Autodesk Inventor part; units mm, degrees
ref_plane "YZ Plane" through (0, 0, 0) normal (1, 0, 0) x (0, 1, 0)
ref_plane "XZ Plane" through (0, 0, 0) normal (0, 1, 0) x (-1, 0, 0)
ref_plane "XY Plane" through (0, 0, 0) normal (0, 0, 1) x (1, 0, 0)
sketch "Эскиз1" plane through (0, 0, 0) normal (0, 1, 0) x (-1, 0, 0)
  line L0 (0, 0) -> (-10, 0)
  line L1 (-10, 0) -> (-10, -11)
  line L2 (-10, -11) -> (0, -11)
  line L3 (0, -11) -> (0, 0)
  dimension "d0" = 10
  dimension "d1" = 11
extrude "Выдавливание1" add sketch "Эскиз1" along normal mid plane 10
sketch "Эскиз2" plane through (0, 0, 0) normal (0, 1, 0) x (-1, 0, 0)
  line L0 (0, -11) -> (0, 0)
  line L1 (0, -5.5) -> (-10, -5.5)
  line L2 (-10, 0) -> (-10, -11)
  line L3 (-1.5, -1.5) -> (-8.5, -1.5)
  line L4 (-8.5, -1.5) -> (-8.5, -9.5)
  line L5 (-8.5, -9.5) -> (-1.5, -9.5)
  line L6 (-1.5, -9.5) -> (-1.5, -1.5)
  line L7 (-1.5, -1.5) -> (-8.5, -9.5) construction
  line L8 (-8.5, -1.5) -> (-1.5, -9.5) construction
  point P0 (-5, -5.5)
  dimension "d4" = 7
  dimension "d5" = 8
extrude "Выдавливание2" cut sketch "Эскиз2" along normal mid plane 7
fillet "Сопряжение1" radius 1 12 edges at (10, 5, -5.5) (5, -5, 0) (5, 5, 0) (0, 5, -5.5) (0, 0, 0) (0, -5, -5.5) (0, 0, -11) (10, 0, -11) (5, 5, -11) (5, -5, -11) (10, -5, -5.5) (10, 0, 0)
sketch "Эскиз3" plane through (0, -4, -1) normal (-1, 0, 0) x (0, 0, 1)
  line L0 (0, 0) -> (0, 8)
  line L1 (0, 4) -> (-9, 4)
  line L2 (-9, 0) -> (-9, 8)
  line L3 (-1, 5) -> (-8, 5)
  line L4 (-8, 5) -> (-8, 3)
  line L5 (-8, 3) -> (-1, 3)
  line L6 (-1, 3) -> (-1, 5)
  line L7 (-1, 5) -> (-8, 3) construction
  line L8 (-8, 5) -> (-1, 3) construction
  point P0 (1, 4)
  point P1 (-4.5, 4)
sketch "Эскиз6" plane through (10, -4, -1) normal (1, 0, 0) x (0, 0, -1)
  line L0 (1, 3) -> (8, 3)
  line L1 (1, 5) -> (1, 3)
  line L2 (8, 5) -> (1, 5)
  line L3 (8, 3) -> (8, 5)
  point P0 (-1, 4)
sketch "Эскиз7" plane through (0, 5, 0) normal (0, 1, 0) x (1, 0, 0)
  line L0 (9, 1) -> (1, 1)
  line L1 (5, 1) -> (5, 10)
  line L2 (9, 10) -> (1, 10)
  line L3 (4, 2) -> (6, 2)
  line L4 (6, 2) -> (6, 9)
  line L5 (6, 9) -> (4, 9)
  line L6 (4, 9) -> (4, 2)
  line L7 (4, 2) -> (6, 9) construction
  line L8 (6, 2) -> (4, 9) construction
  point P0 (0, 0)
  point P1 (5, 5.5)
sketch "Эскиз8" plane through (0, -5, 0) normal (0, -1, 0) x (1, 0, 0)
  line L0 (4, -9) -> (4, -2)
  line L1 (6, -9) -> (4, -9)
  line L2 (6, -2) -> (6, -9)
  line L3 (4, -2) -> (6, -2)
  point P0 (0, 0)
extrude "Выдавливание5" cut sketch "Эскиз7" against normal blind 0.5
extrude "Выдавливание6" cut sketch "Эскиз3" against normal blind 0.5
extrude "Выдавливание7" cut sketch "Эскиз8" against normal blind 0.5
extrude "Выдавливание8" cut sketch "Эскиз6" against normal blind 0.5
properties part number "cube"
The listing builds one solid part. Answer for the finished solid, in the listing's coordinates (mm). A direction names the side the tool comes from. Give positions to 0.01 mm unless a question says otherwise; leave off trailing zeros. Write each loop counter-clockwise with the first axis right and the second up, starting at its lowest first coordinate (ties: lowest second). Pieces come first, ordered by that corner, then holes. Notation, with made-up numbers: (21, 43.5) - (28, 43.5) arc R29 cw to (28, 77.5) - close; hole circle Ø10 at (-20, 39). An arc over 180 degrees is marked (long way). Use one line per item in the form item = value. Start each with the question number.
1) The mould has two halves that part along Z. Classify faces 1 (the face through (0.285, -4.699, -5.437)), 2 (the face through (0.5, 0, -6)), 3 (the face through (9.699, 0.056, -0.285)), 4 (the face through (5, 0, -11)): pulls with the +Z half, pulls with the -Z half, needs draft (parallel to the pull), parting line crosses it, or undercut.
2) Consider line 1 along X through (y, z) = (1, -9.25); line 2 along Z through (x, y) = (4, -2); line 3 along Y through (x, z) = (7.25, -5.5). Determine where each line is inside the solid, lowest interval first. Write a range as from..to.
3) Flat-ended cylindrical pins translate along their axes: pin 1 Ø2 at (x, z) = (4.5, -7) entering from -Y; pin 2 Ø0.6 at (x, z) = (0.5, -4) entering from +Y. Find the tip coordinate at first contact, or state that the pin passes through.
4) Find section C-C on z = -3.5. Determine the outline of the cut face in (x, y), plus the area to 3 significant figures.
5) A tool of negligible diameter and unlimited length cuts with its end or side. For faces 5 (the face through (4.944, 4.715, -10.699)), 6 (the face through (5, 4.5, -6)), 7 (the face through (5, -3.5, -5)), 8 (the face through (9.715, -4.699, -5.563)), 9 (the face through (5, -4.5, -5)), from which of +Z, -Z, +X, -X, +Y, -Y can it reach the whole face along a straight path? Write none if from no direction.
6) Find section D-D on x = 5.5. Determine the outline of the cut face in (y, z).
7) Find section B-B on x = 6.5. Determine the outline of the cut face in (y, z).
8) Find section A-A on y = -0.25. Determine the outline of the cut face in (x, z), plus the area to 3 significant figures.
Geometry results:
q1.face_1 = needs draft
q1.face_2 = undercut
q1.face_3 = pulls with the +Z half
q1.face_4 = pulls with the -Z half
q2.line_1 = 0..1.5, 8.5..10
q2.line_2 = -11..-9.5, -1.5..0
q2.line_3 = -5..-3.5, 3.5..5
q3.pin_1 = -5
q3.pin_2 = 4.98
q4.outline = (0, -4) arc R1 ccw to (1, -5) - (4, -5) - (4, -4.5) - (6, -4.5) - (6, -5) - (9, -5) arc R1 ccw to (10, -4) - (10, -1) - (9.5, -1) - (9.5, 1) - (10, 1) - (10, 4) arc R1 ccw to (9, 5) - (6, 5) - (6, 4.5) - (4, 4.5) - (4, 5) - (1, 5) arc R1 ccw to (0, 4) - (0, 1) - (0.5, 1) - (0.5, -1) - (0, -1) - close; hole (1.5, -3.5) - (8.5, -3.5) - (8.5, 3.5) - (1.5, 3.5) - close
q4.area = 46.1 mm2
q5.face_5 = -Z, +X, -X, +Y
q5.face_6 = +Y
q5.face_7 = none
q5.face_8 = +Z, -Z, +X, -Y
q5.face_9 = -Y
q6.outline = (-5, -10) arc R1 ccw to (-4, -11) - (4, -11) arc R1 ccw to (5, -10) - (5, -9) - (4.5, -9) - (4.5, -2) - (5, -2) - (5, -1) arc R1 ccw to (4, 0) - (-4, 0) arc R1 ccw to (-5, -1) - (-5, -2) - (-4.5, -2) - (-4.5, -9) - (-5, -9) - close; hole (-3.5, -9.5) - (3.5, -9.5) - (3.5, -1.5) - (-3.5, -1.5) - close
q7.outline = (-5, -10) arc R1 ccw to (-4, -11) - (4, -11) arc R1 ccw to (5, -10) - (5, -1) arc R1 ccw to (4, 0) - (-4, 0) arc R1 ccw to (-5, -1) - close; hole (-3.5, -9.5) - (3.5, -9.5) - (3.5, -1.5) - (-3.5, -1.5) - close
q8.outline = (0, -10) arc R1 ccw to (1, -11) - (9, -11) arc R1 ccw to (10, -10) - (10, -9) - (9.5, -9) - (9.5, -2) - (10, -2) - (10, -1) arc R1 ccw to (9, 0) - (1, 0) arc R1 ccw to (0, -1) - (0, -2) - (0.5, -2) - (0.5, -9) - (0, -9) - close; hole (1.5, -9.5) - (8.5, -9.5) - (8.5, -1.5) - (1.5, -1.5) - close
q8.area = 46.1 mm2
